from build123d import *

# Parameters (mm, degrees)
BOSS_EXTRUDE1_DEPTH = 80
CHAMFER1_SIZE       = 12
CHAMFER1_SIZE2      = 21
CHAMFER2_SIZE       = 12
CHAMFER2_SIZE2      = 21
SKETCH2_R           = 9
CUT_EXTRUDE1_DEPTH  = 80
BOSS_EXTRUDE2_DEPTH = 36


with BuildPart() as part:
    # Sketch1 → Boss-Extrude1 (new body)
    with BuildSketch(Plane(origin=(0, 0, 0), x_dir=(0, 0, -1), z_dir=(1, 0, 0))):
        Polygon((-44.171875, 0), (-44.171875, 36), (-10.171875, 82), (21.828125, 82), (21.828125, 0), align=None)
    extrude(amount=-BOSS_EXTRUDE1_DEPTH)

    # Chamfer1
    chamfer1_edges = [part.edges().sort_by_distance(p)[0] for p in [
        (0, 82, -5.828125),
    ]]
    chamfer1_side = [part.faces().sort_by_distance(p)[0] for p in [
        (-40, 82, -5.828125),
    ]]
    chamfer(chamfer1_edges, length=CHAMFER1_SIZE, length2=CHAMFER1_SIZE2, reference=chamfer1_side[0])

    # Chamfer2
    chamfer2_edges = [part.edges().sort_by_distance(p)[0] for p in [
        (-80, 82, -5.828125),
    ]]
    chamfer2_side = [part.faces().sort_by_distance(p)[0] for p in [
        (-46, 82, -5.828125),
    ]]
    chamfer(chamfer2_edges, length=CHAMFER2_SIZE, length2=CHAMFER2_SIZE2, reference=chamfer2_side[0])

    # Sketch2 → Cut-Extrude1 (cut)
    with BuildSketch(Plane(origin=(0, 82, 0), x_dir=(1, 0, 0), z_dir=(0, 1, 0))):
        with Locations(Location((-42.415623136, 6.828125, 0), (0, 0, 270))):
            Circle(SKETCH2_R)
    extrude(amount=-CUT_EXTRUDE1_DEPTH, mode=Mode.SUBTRACT)

    # Sketch3 → Boss-Extrude2 (add)
    with BuildSketch(Plane.XZ):
        with BuildLine():
            Line((-65, 128.171875), (-65, 44.171875))
            Line((-65, 44.171875), (-15, 44.171875))
            Line((-15, 44.171875), (-15, 128.171875))
            Line((-15, 128.171875), (-30, 128.171875))
            Line((-30, 128.171875), (-30, 83.171875))
            ThreePointArc((-30, 83.171875), (-40, 73.171875), (-50, 83.171875))
            Line((-50, 83.171875), (-50, 128.171875))
            Line((-50, 128.171875), (-65, 128.171875))
        make_face()
    extrude(amount=-BOSS_EXTRUDE2_DEPTH)


solid = part.part
Check sheet for the modelled part. Datum: model origin and axes. Units: mm. A direction names the side the tool comes from. Give positions to 0.01 mm unless a question says otherwise; leave off trailing zeros. Loops run counter-clockwise (first coordinate to the right, second up) from the corner with the lowest first, then second, coordinate; pieces in that order, holes last. Notation, with made-up numbers: M 88,23 L 141,23 A23 ccw 141,32 Z; hole C 32,79 d9. An arc over 180 degrees is marked long. Return JSON: item names as keys, results as strings. Group by question number.
1. Cross-section at B-B on x = -26. Record the boundary of the cut face in (y, z), plus the area to 3 significant figures.
2. Cross-section at A-A on z = 114. Record the boundary of the cut face in (x, y), plus the area to 3 significant figures.
3. Thickness scan on L1, parallel to Y at x = -63, z = 61.5; L2, parallel to Z at x = -4, y = 26; L3, parallel to Z at x = -36.5, y = 60. Record the ranges inside material, lowest first.
4. Cross-section at C-C on y = 41.5. Record the boundary of the cut face in (x, z), plus the area to 3 significant figures.
5. Tool access check on faces 4 (the flat face through (-65, 18, 87)), 5 (the flat face through (-51, 36, 87)), 6 (the flat face through (-30, 18, 106)), 7 (the flat face through (-80, 31, 11)), 8 (the cylindrical face through (-50.4, 42.56, -2.675)). Record the directions out of +Z, -Z, +X, -X, +Y, -Y that give a thin tool (end or side, any length) a straight path to the whole face; none if there is none.
6. Go/stop test with flat-tipped pins: pin 1 (25 mm diameter, centred on x = -50, z = 86, fed in from +Y); pin 2 (1 mm diameter, centred on x = -48.5, y = 58, fed in from +Z); pin 3 (18 mm diameter, centred on y = 25.5, z = 102.5, fed in from +X); pin 4 (8 mm diameter, centred on y = 43.5, z = 79.5, fed in from -X). Record where each tip stops, or that it passes through.
7. Cross-section at D-D on z = 60.5. Record the boundary of the cut face in (x, y).
8. Mould release check, pull along X, two halves, no side actions. Record for faces 1 (the flat face through (-15, 18, 86)), 2 (the flat face through (-39.44, 58.68, 27.41)), 3 (the flat face through (-50, 18, 105)): released by +X, released by -X, zero draft, split by the parting line, or undercut.
Return value:
{
 "1": {"outline": "M 0,-21.83 L 82,-21.83 L 82,10.17 L 36,44.17 L 36,128.17 L 0,128.17 Z", "area": "7,650 mm^2"},
 "2": {"outline": "M -65,0 L -50,0 L -50,36 L -65,36 Z; M -30,0 L -15,0 L -15,36 L -30,36 Z", "area": "1,080 mm^2"},
 "3": {"L1": "0 to 36", "L2": "-21.83 to 44.17", "L3": "-21.83 to -13.61, -0.05 to 26.43"},
 "4": {"outline": "M -80,-21.83 L 0,-21.83 L 0,40.11 L -80,40.11 Z; hole C -42.42,-6.83 d18", "area": "4,700 mm^2"},
 "5": {"face 4": "+Z, -X, +Y, -Y", "face 5": "+Z, +X, -X, +Y", "face 6": "+Z, +Y, -Y", "face 7": "+Z, -Z, -X, +Y, -Y", "face 8": "+Y"},
 "6": {"pin 1": "y = 36", "pin 2": "z = 28.28", "pin 3": "x = -15", "pin 4": "through"},
 "7": {"outline": "M -65,0 L -15,0 L -15,36 L -65,36 Z"},
 "8": {"face 1": "released by +X", "face 2": "zero draft", "face 3": "undercut"}
}
